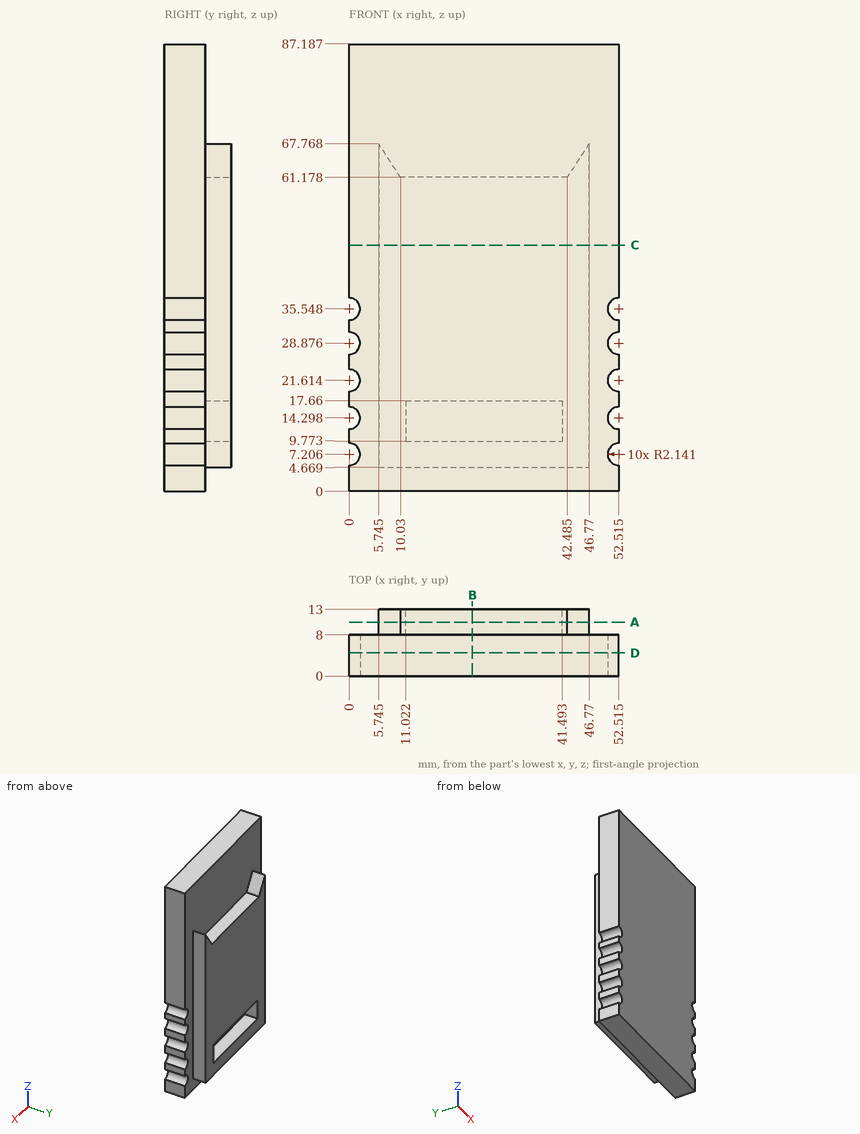
Check sheet for the drawn part. Datum: minimum x, y, z corner. Units: mm. Give positions to 0.01 mm unless a question says otherwise; leave off trailing zeros. Write each loop counter-clockwise with the first axis right and the second up, starting at its lowest first coordinate (ties: lowest second). Pieces come first, ordered by that corner, then holes. Notation, with made-up numbers: M 28,-8.75 L 51,-8.75 A3 ccw 51,-3.75 Z; hole C 58,87.25 d7. An arc over 180 degrees is marked long. One line per question, with ' | ' between items.
1. Cross-section at D-D (y = 4.5). Enter the section's corners in (x, z) (1 decimal).
Ans:
outline: M 0,0 L 52.5,0 L 52.5,5.1 A2.1 cw 52.5,9.3 L 52.5,12.2 A2.1 cw 52.5,16.4 L 52.5,19.5 A2.1 cw 52.5,23.8 L 52.5,26.7 A2.1 cw 52.5,31 L 52.5,33.4 A2.1 cw 52.5,37.7 L 52.5,87.2 L 0,87.2 L 0,37.7 A2.1 cw 0,33.4 L 0,31 A2.1 cw 0,26.7 L 0,23.8 A2.1 cw 0,19.5 L 0,16.4 A2.1 cw 0,12.2 L 0,9.3 A2.1 cw 0,5.1 Z
2. Gauge pin test, flat ends, axial feed: pin 1 (4 mm diameter, centred on x = 21, z = 12.5, fed in from +Y); pin 2 (5.5 mm diameter, centred on x = 34, y = 11.5, fed in from -Z); pin 3 (1.5 mm diameter, centred on y = 9.5, z = 14.5, fed in from +X). Record the tip position at first contact, or that the pin passes through.
Ans:
pin 1: y = 8 | pin 2: z = 4.67 | pin 3: x = 46.77
3. Scan lines: line 1 along Z through (x, y) = (21, 10); line 2 along X through (y, z) = (10.75, 12.5) (1 decimal); line 3 along Y through (x, z) = (45, 77). Record each from-to range of solid material in increasing order. Write a range as from..to.
Ans:
line 1: 4.67..9.77, 17.66..61.18 | line 2: 5.7..11, 41.5..46.8 | line 3: 0..8
4. Cross-section at B-B (x = 24). Enter the section's corners in (y, z).
Ans:
outline: M 0,0 L 8,0 L 8,4.67 L 13,4.67 L 13,9.77 L 8,9.77 L 8,17.66 L 13,17.66 L 13,61.18 L 8,61.18 L 8,87.19 L 0,87.19 Z
5. Cross-section at A-A (y = 10.5). Enter the section's corners in (x, z) (1 decimal).
Ans:
outline: M 5.7,4.7 L 46.8,4.7 L 46.8,67.8 L 42.5,61.2 L 10,61.2 L 5.7,67.8 Z; hole M 11,9.8 L 41.5,9.8 L 41.5,17.7 L 11,17.7 Z
6. Cross-section at C-C (z = 48). Enter the section's corners in (x, y) (1 decimal), plus the area to 3 significant figures.
Ans:
outline: M 0,0 L 52.5,0 L 52.5,8 L 46.8,8 L 46.8,13 L 5.7,13 L 5.7,8 L 0,8 Z | area: 625 mm2
